Here's the drawing with two shaded views (mm, measured from the low corner). I have some questions. Round coordinates to 2 decimals unless told otherwise and drop trailing zeros. Loops run counter-clockwise (first coordinate to the right, second up) from the corner with the lowest first, then second, coordinate; pieces in that order, holes last.
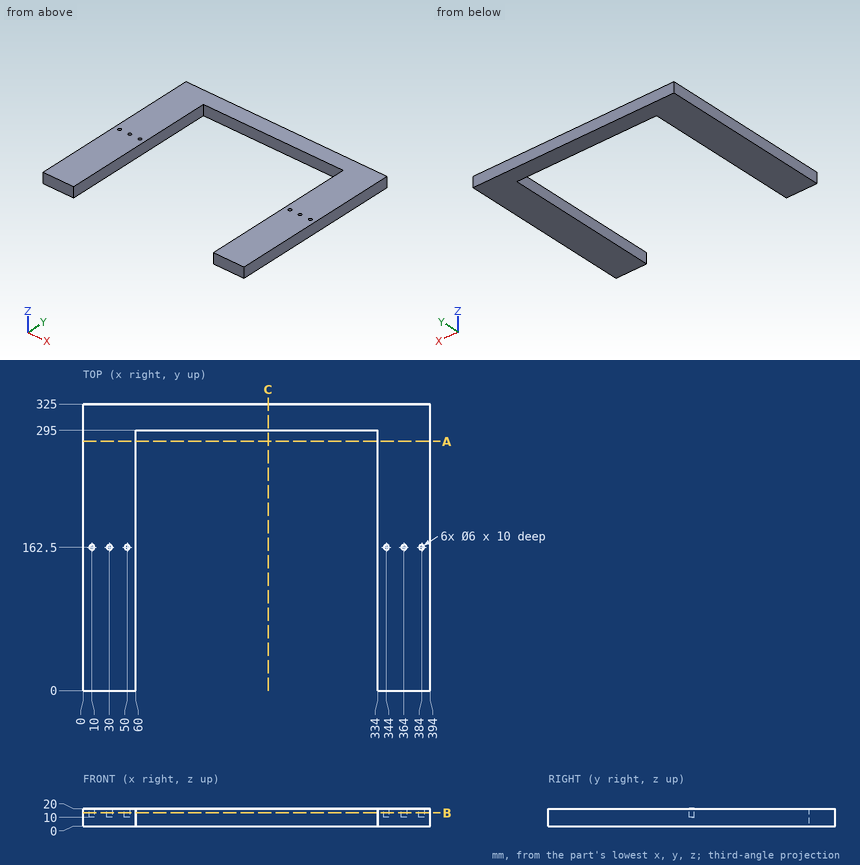
Item 1: If we section it at A-A, the plane y = 282.5: Please give me the cut outline in (x, z), then the cut area to 3 significant figures.
Results list:
outline: (0, 0) - (60, 0) - (60, 20) - (0, 20) - close; (334, 0) - (394, 0) - (394, 20) - (334, 20) - close
area: 2,400 mm2
Item 2: Will these pins go through, and if not, where does the flat tip stop? pin 1 (3 mm diameter, centred on x = 307, z = 15.5, fed in from -Y); pin 2 (1.8 mm diameter, centred on x = 344.5, y = 163, fed in from +Z).
Results list:
pin 1: stops at y = 295
pin 2: stops at z = 10
Item 3: If we section it at C-C, the plane x = 210: Please give me the cut outline in (y, z), then the cut area to 3 significant figures.
Results list:
outline: (295, 0) - (325, 0) - (325, 20) - (295, 20) - close
area: 600 mm2
Item 4: If we section it at B-B, the plane z = 15: Please give me the cut outline in (x, y), then the cut area to 3 significant figures.
Results list:
outline: (0, 0) - (60, 0) - (60, 295) - (334, 295) - (334, 0) - (394, 0) - (394, 325) - (0, 325) - close; hole circle Ø6 at (10, 162.5); hole circle Ø6 at (30, 162.5); hole circle Ø6 at (50, 162.5); hole circle Ø6 at (344, 162.5); hole circle Ø6 at (364, 162.5); hole circle Ø6 at (384, 162.5)
area: 47,100 mm2
Item 5: If I drill on line 1 along Y through (x, z) = (384, 12); line 2 along X through (y, z) = (74, 12.75); line 3 along Y through (x, z) = (227, 1.5), over which ranges is the centre line in solid material (lowest first)?
Results list:
line 1: y = 0 to 159.5, 165.5 to 325
line 2: x = 0 to 60, 334 to 394
line 3: y = 295 to 325
